```python
from build123d import *

# Parameters (mm, degrees)
SKETCH2_W           = 57.15
SKETCH2_H           = 57.15
SKETCH2_R           = 12.7
BOSS_EXTRUDE2_DEPTH = 4.826
SKETCH2_4_R         = 3.175
CUT_EXTRUDE4_DEPTH  = 5.826
CIRPATTERN1_COUNT   = 8


with BuildPart() as part:
    # Sketch2 → Boss-Extrude2 (new body)
    with BuildSketch(Plane(origin=(0, 0, 0), x_dir=(0, 0, -1), z_dir=(1, 0, 0))):
        with Locations((-19.436862591, 6.909929069)):
            Rectangle(SKETCH2_W, SKETCH2_H)
        with Locations((-19.436862591, 10.084929069)):
            Circle(SKETCH2_R, mode=Mode.SUBTRACT)
    extrude(amount=BOSS_EXTRUDE2_DEPTH)

    # Sketch2_4 → Cut-Extrude4 (cut, through all)
    with BuildSketch(Plane(origin=(0, 0, 0), x_dir=(0, 0, -1), z_dir=(1, 0, 0))):
        with Locations((-19.436862591, 29.134929069)):
            Circle(SKETCH2_4_R)
    cut_extrude4 = extrude(amount=CUT_EXTRUDE4_DEPTH, mode=Mode.SUBTRACT)

    # CirPattern1: Cut-Extrude4 ×8 about axis
    cirpattern1_axis = Axis((0, 10.084929069, 19.436862591), (1, 0, 0))
    for i in range(1, CIRPATTERN1_COUNT):
        add(cut_extrude4.rotate(cirpattern1_axis, i * 360 / CIRPATTERN1_COUNT), mode=Mode.SUBTRACT)


solid = part.part
```
Input: part model. Units: mm. Frame: model coordinates. Give positions to 0.01 mm unless a question says otherwise; leave off trailing zeros. Order: outer loops, then holes, each group sorted by start corner. A loop starts at its lowest first (then second) coordinate and runs counter-clockwise, first axis right, second up. Notation, with made-up numbers: (26.5, 88) - (83.5, 88) arc R18 cw to (83.5, 115) - close; hole circle Ø1 at (84, 69.25). An arc over 180 degrees is marked (long way). Use a Markdown table: item, result.
(1) Draft query along Y for faces 1 (the flat face through (2, 7, 48.012)), 2 (the flat face through (2, 35.485, 20)), 3 (the cylindrical face through (2.379, 20.528, 6.922)), 4 (the cylindrical face through (2.38, -5.32, 3.45)). Return one class per face: released by +Y, released by -Y, zero draft, split by the parting line, or undercut.
Computed values:
| item | result |
|---|---|
| face 1 | zero draft |
| face 2 | released by +Y |
| face 3 | undercut |
| face 4 | undercut |
(2) Line query: line 1 (Z direction, x = 1.85, y = -3.5); line 2 (Y direction, x = 2.4, z = 33); line 3 (Z direction, x = 1.2, y = 23). Output: solid intervals per line, ascending. Write a range as from..to.
Computed values:
| item | result |
|---|---|
| line 1 | z = -9.14..2.79, 9.14..29.73, 36.08..48.01 |
| line 2 | y = -21.67..-6.56, -0.21..20.38, 26.73..35.48 |
| line 3 | z = -9.14..2.84, 9.09..29.78, 36.03..48.01 |
(3) Section query A-A (y = 3). Output: boundary loops of the cut face in (x, z), then the cut area to 3 significant figures.
Computed values:
| item | result |
|---|---|
| outline | (0, -9.14) - (4.83, -9.14) - (4.83, 8.9) - (0, 8.9) - close; (0, 29.98) - (4.83, 29.98) - (4.83, 48.01) - (0, 48.01) - close |
| area | 174 mm2 |
(4) Section query C-C (x = 3.95). State how many separate pieces and enclosed holes the cut face has, then the cut area to 3 significant figures.
Computed values:
| item | result |
|---|---|
| separate pieces | 1 |
| enclosed holes | 9 |
| area | 2,510 mm2 |
(5) Section query B-B (z = 37.5). Output: boundary loops of the cut face in (x, y).
Computed values:
| item | result |
|---|---|
| outline | (0, -21.67) - (4.83, -21.67) - (4.83, 7.07) - (0, 7.07) - close; (0, 13.1) - (4.83, 13.1) - (4.83, 35.48) - (0, 35.48) - close |
